from build123d import *

# Parameters (mm, degrees)
SKETCH_1_W          = 90
SKETCH_1_H          = 28
SKETCH_1_R          = 4.25
SKETCH_1_R_2        = 2
EXTRUDE_1_DEPTH     = 3
CUT_EXTRUDE_1_REACH = 49.223
SKETCH_3_R          = 2.25
SKETCH_4_W          = 20
SKETCH_4_H          = 25
EXTRUDE_3_DEPTH     = 3
FILLET_6_R          = 18.5
FILLET_9_R          = 10
EXTRUDE_4_DEPTH     = 3
FILLET_11_RADIUS    = 14
FILLET_11_LENGTH    = 3


with BuildPart() as part:
    # 草图1 → 凸台-拉伸1 (new body)
    with BuildSketch(Plane(origin=(0, 0, 0), x_dir=(1, 0, 0), z_dir=(0, 1, 0))):
        Rectangle(SKETCH_1_W, SKETCH_1_H)
        with Locations(Location((17.5, 0, 0), (0, 0, 270))):
            Circle(SKETCH_1_R, mode=Mode.SUBTRACT)
        with Locations(Location((-32.5, 0, 0), (0, 0, 270))):
            Circle(SKETCH_1_R_2, mode=Mode.SUBTRACT)
    extrude(amount=EXTRUDE_1_DEPTH)

    # 草图3 → 切除-拉伸1 (cut, up to next)
    with BuildSketch(Plane(origin=(0, 3, 0), x_dir=(1, 0, 0), z_dir=(0, 1, 0)), mode=Mode.PRIVATE) as cut_extrude_1_sk1:
        with Locations(Location((36, 0, 0), (0, 0, 270))):
            Circle(SKETCH_3_R)
    cut_extrude_1_tool1 = extrude(cut_extrude_1_sk1.sketch, amount=-CUT_EXTRUDE_1_REACH, mode=Mode.PRIVATE) & part.part
    # 草图3 → 切除-拉伸1 (cut, up to next)
    with BuildSketch(Plane(origin=(0, 3, 0), x_dir=(1, 0, 0), z_dir=(0, 1, 0)), mode=Mode.PRIVATE) as cut_extrude_1_sk2:
        with Locations(Location((-1, 0, 0), (0, 0, 270))):
            Circle(SKETCH_3_R)
    cut_extrude_1_tool2 = extrude(cut_extrude_1_sk2.sketch, amount=-CUT_EXTRUDE_1_REACH, mode=Mode.PRIVATE) & part.part
    add(cut_extrude_1_tool1.solids().sort_by_distance((36, 3, 0))[0], mode=Mode.SUBTRACT)
    add(cut_extrude_1_tool2.solids().sort_by_distance((-1, 3, 0))[0], mode=Mode.SUBTRACT)

    # 草图4 → 凸台-拉伸3 (add)
    with BuildSketch(Plane(origin=(0, 3, 0), x_dir=(1, 0, 0), z_dir=(0, 1, 0))):
        with Locations((-16.5, 26.5)):
            Rectangle(SKETCH_4_W, SKETCH_4_H)
    extrude(amount=-EXTRUDE_3_DEPTH)

    # 圆角6
    fillet_6_edges = [part.edges().sort_by_distance(p)[0] for p in [
        (-26.5, 1.5, -14),
        (-6.5, 1.5, -14),
    ]]
    fillet(fillet_6_edges, radius=FILLET_6_R - 0.0001)  # a hair under: the kernel refuses the full size

    # 圆角9
    fillet_9_edges = [part.edges().sort_by_distance(p)[0] for p in [
        (-6.5, 1.5, -39),
        (-26.5, 1.5, -39),
    ]]
    fillet(fillet_9_edges, radius=FILLET_9_R)

    # 草图6 → 凸台-拉伸4 (add)
    with BuildSketch(Plane(origin=(0, 3, 0), x_dir=(1, 0, 0), z_dir=(0, 1, 0))):
        with BuildLine():
            Line((-45, -14), (-45, 14))
            ThreePointArc((-45, 14), (-59, 0), (-45, -14))
        make_face()
    extrude(amount=-EXTRUDE_4_DEPTH)

    # 圆角11: full round fillet: the end face becomes a half cylinder, R = half its width
    fillet_11_face = Plane((45, 1.5, 0), x_dir=(0, -1, 0), z_dir=(1, 0, 0))  # on the end face: x along it, z out of the body
    fillet_11_slab = fillet_11_face.offset(-FILLET_11_RADIUS / 2) * Box(FILLET_11_LENGTH, 2 * FILLET_11_RADIUS, FILLET_11_RADIUS, mode=Mode.PRIVATE)  # the body's end, R deep
    fillet_11_round = Plane((31, 1.5, 0), x_dir=(1, 0, 0), z_dir=(0, -1, 0)) * Cylinder(FILLET_11_RADIUS, FILLET_11_LENGTH, mode=Mode.PRIVATE)  # its axis R under the face
    add(fillet_11_slab - fillet_11_round, mode=Mode.SUBTRACT)


solid = part.part
Work out the finished part from the listing and answer in its coordinate system (mm). Round coordinates to 2 decimals unless told otherwise and drop trailing zeros. Loops run counter-clockwise (first coordinate to the right, second up) from the corner with the lowest first, then second, coordinate; pieces in that order, holes last. Notation, with made-up numbers: (14.25, 57) -> (70.25, 57) arc R4 cw to (70.25, 63) -> close; hole circle Ø6 at (-25, 40.5). An arc over 180 degrees is marked (long way). Use one line per item in the form item = value.
(1) For a pull along X with two mould halves and no side action, classify faces 1 (the cylindrical face through (38.23, 1.52, -0.29)), 2 (the flat face through (21, 1, -14)), 3 (the cylindrical face through (-59, 2, 0)), 4 (the cylindrical face through (1.23, 1.52, -0.29)) as released by +X, released by -X, zero draft, split by the parting line, or undercut.
Answer list:
face_1 = undercut
face_2 = zero draft
face_3 = released by -X
face_4 = undercut
(2) A flat-ended cylindrical pin translates along its axis: P1, Ø1.5, axis at x = 15, y = 2.5, coming from the -Z side. Find the tip coordinate at first contact, or state that the pin passes through.
Answer list:
P1 = -14
(3) Find section C-C on x = -32.5. Give the vertices of the cut face in (y, z), then the cut area to 3 significant figures.
Answer list:
outline = (0, -18.86) -> (3, -18.86) -> (3, -2) -> (0, -2) -> close; (0, 2) -> (3, 2) -> (3, 14) -> (0, 14) -> close
area = 86.6 mm2
(4) Straight lines are drawn through the part: line 1 (X direction, y = 0.65, z = 0); line 2 (Z direction, x = 18.5, y = 1.15); line 3 (X direction, y = 1.3, z = -4.5). For each, find the intervals that lie inside material, in ascending order.
Answer list:
line_1 = -59 to -34.5, -30.5 to -3.25, 1.25 to 13.25, 21.75 to 33.75, 38.25 to 45
line_2 = -14 to -4.13, 4.13 to 14
line_3 = -58.26 to 44.26
(5) Find section A-A on x = 17.5. Give the vertices of the cut face in (y, z).
Answer list:
outline = (0, -14) -> (3, -14) -> (3, -4.25) -> (0, -4.25) -> close; (0, 4.25) -> (3, 4.25) -> (3, 14) -> (0, 14) -> close
(6) Find section B-B on z = 0. Give the vertices of the cut face in (x, y), then the cut area to 4 significant figures.
Answer list:
outline = (-59, 0) -> (-34.5, 0) -> (-34.5, 3) -> (-59, 3) -> close; (-30.5, 0) -> (-3.25, 0) -> (-3.25, 3) -> (-30.5, 3) -> close; (1.25, 0) -> (13.25, 0) -> (13.25, 3) -> (1.25, 3) -> close; (21.75, 0) -> (33.75, 0) -> (33.75, 3) -> (21.75, 3) -> close; (38.25, 0) -> (45, 0) -> (45, 3) -> (38.25, 3) -> close
area = 247.5 mm2
(7) Find section D-D on y = 2.2. Give the number of separate pieces and of enclosed holes in the cut face, then the cut area to 3 significant figures.
Answer list:
separate_pieces = 1
enclosed_holes = 4
area = 3,250 mm2
